Input: dimensioned drawing with shaded views. Units: mm. Origin: part minimum x, y, z. Give positions to 0.01 mm unless a question says otherwise; leave off trailing zeros. Write each loop counter-clockwise with the first axis right and the second up, starting at its lowest first coordinate (ties: lowest second). Pieces come first, ordered by that corner, then holes.
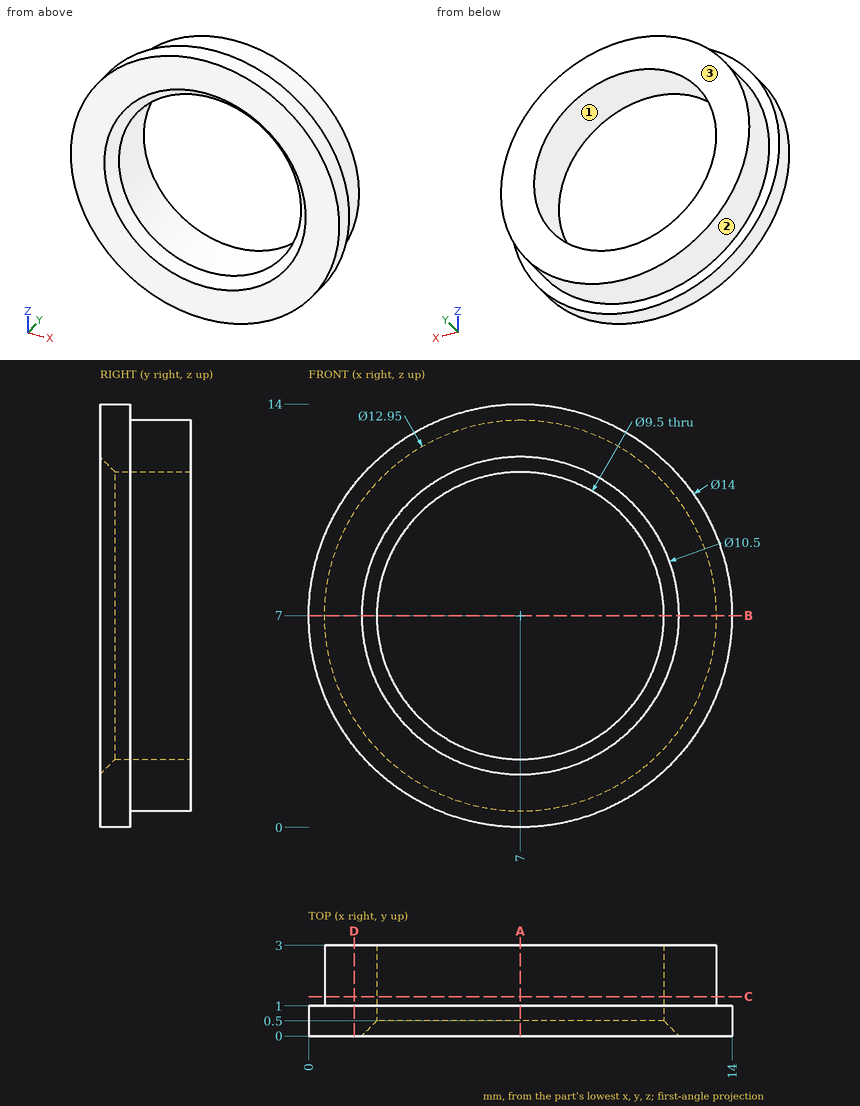
1. Cut plane D-D, the plane x = 1.5. Return the cut outline in (y, z).
2. Cut plane B-B, the plane z = 7. Return the cut outline in (x, y) (3 decimals), then the cut area to 4 significant figures.
3. Mould query, pull axis Z, two halves, no side actions, for the marked faces 1, 2 and 3. Classes: +Z half, -Z half, draft (parallel to the pull), parting line (faces both ways), or undercut.
4. Contact query for flat-ended pins moving along their axis: P1, Ø6, axis at x = 7, z = 5, coming from the -Y side; P2, Ø1.5, axis at y = 1.5, z = 2, coming from the +X side. Output: stop coordinate, or through.
5. Cut plane C-C, the plane y = 1.3. Return the cut outline in (x, z) (3 decimals).
6. Line query: L1, parallel to X at y = 1.65, z = 7 (3 decimals); L2, parallel to X at y = 0.7, z = 6; L3, parallel to Z at x = 4.5, y = 1.3. Output: solid intervals per line, ascending.
7. Cut plane A-A, the plane x = 7. Return the cut outline in (y, z) (3 decimals).
Response values:
1. outline: (0, 2.67) - (1, 2.67) - (1, 3.58) - (3, 3.58) - (3, 10.42) - (1, 10.42) - (1, 11.33) - (0, 11.33) - close
2. outline: (0, 0) - (1.75, 0) - (2.25, 0.5) - (2.25, 3) - (0.525, 3) - (0.525, 1) - (0, 1) - close; (11.75, 0.5) - (12.25, 0) - (14, 0) - (14, 1) - (13.475, 1) - (13.475, 3) - (11.75, 3) - close
2. area: 11.15 mm2
3. face 1: undercut
3. face 2: parting line
3. face 3: draft
4. P1: stops at y = 0.25
4. P2: stops at x = 12.41
5. outline: circle Ø12.95 at (7, 7); hole circle Ø9.5 at (7, 7)
6. L1: x = 0.525 to 2.25, 11.75 to 13.475
6. L2: x = 0.07 to 2.36, 11.64 to 13.93
6. L3: z = 1.03 to 2.96, 11.04 to 12.97
7. outline: (0, 0) - (1, 0) - (1, 0.525) - (3, 0.525) - (3, 2.25) - (0.5, 2.25) - (0, 1.75) - close; (0, 12.25) - (0.5, 11.75) - (3, 11.75) - (3, 13.475) - (1, 13.475) - (1, 14) - (0, 14) - close
